```python
from build123d import *

# Parameters (mm, degrees)
SKETCH_3_R               = 5
CUT_EXTRUDE_2_DEPTH      = 151.643619181
PATTERN_CIRCULAR_1_COUNT = 4
CHAMFER_1_SIZE           = 0.5
CHAMFER_2_SIZE           = 0.5


with BuildPart() as part:
    # 草图1 → 旋转1 (revolve)
    with BuildSketch(Plane.XY, mode=Mode.PRIVATE) as revolve_1_sk:
        Polygon((0, 57.5), (0, 72.5), (38, 72.5), (38, 102.5), (53, 102.5), (53, 78), (79, 78), (79, 67.5), (63.5, 67.5), (63.5, 47.5), (58, 47.5), (58, 52.5), (45, 52.5), (45, 57.5), (5, 57.5), (5, 58.5), (3, 58.5), (3, 57.5), align=None)
    revolve(revolve_1_sk.sketch.rotate(Axis((0, 0, 0), (1, 0, 0)), 90), axis=Axis((0, 0, 0), (1, 0, 0)))

    # 草图3 → 切除-拉伸2 (cut, through all)
    with BuildSketch(Plane.ZY.offset(-38)):
        with Locations((0, 92.5)):
            Circle(SKETCH_3_R)
        with Locations((54.370135837, 74.83407198)):
            Circle(SKETCH_3_R)
        with Locations((87.972727757, 28.58407198)):
            Circle(SKETCH_3_R)
        with Locations((87.972727757, -28.58407198)):
            Circle(SKETCH_3_R)
        with Locations((54.370135837, -74.83407198)):
            Circle(SKETCH_3_R)
        with Locations((0, -92.5)):
            Circle(SKETCH_3_R)
        with Locations((-54.370135837, -74.83407198)):
            Circle(SKETCH_3_R)
        with Locations((-87.972727757, -28.58407198)):
            Circle(SKETCH_3_R)
        with Locations((-87.972727757, 28.58407198)):
            Circle(SKETCH_3_R)
        with Locations((-54.370135837, 74.83407198)):
            Circle(SKETCH_3_R)
    extrude(amount=-CUT_EXTRUDE_2_DEPTH, mode=Mode.SUBTRACT)

    # 草图5 → Ø5.0 (5) 直径孔1 (revolve, cut)
    with BuildSketch(Plane.ZX.offset(65)):
        Polygon((0, 0), (0, 16.502151548), (2.5, 15), (2.5, 0), align=None)
    hole_wizard_5_0_5_1 = revolve(axis=Axis((-6.35, 65, 0), (1, 0, 0)), mode=Mode.SUBTRACT)

    # 阵列(圆周)1: Ø5.0 (5) 直径孔1 ×4 about axis
    pattern_circular_1_axis = Axis((0, 0, 0), (1, 0, 0))
    for i in range(1, PATTERN_CIRCULAR_1_COUNT):
        add(hole_wizard_5_0_5_1.rotate(pattern_circular_1_axis, i * 360 / PATTERN_CIRCULAR_1_COUNT), mode=Mode.SUBTRACT)

    # 倒角1
    chamfer_1_edges = [part.edges().sort_by_distance(p)[0] for p in [
        (38, 0, -102.5),
        (53, 0, -102.5),
        (79, 0, -78),
        (79, 0, -67.5),
        (63.5, 0, -47.5),
        (58, 0, -47.5),
        (45, 0, -52.5),
        (0, 0, -72.5),
    ]]
    chamfer(chamfer_1_edges, length=CHAMFER_1_SIZE)

    # 倒角2
    chamfer_2_edges = [part.edges().sort_by_distance(p)[0] for p in [
        (0, -2.5, -65),
        (53, 92.5, -5),
        (38, 92.5, -5),
        (53, 74.83407198, -59.370135837),
        (38, 74.83407198, -59.370135837),
        (53, 28.58407198, -92.972727757),
        (38, 28.58407198, -92.972727757),
        (53, -28.58407198, -92.972727757),
        (38, -28.58407198, -92.972727757),
        (53, -74.83407198, -59.370135837),
        (38, -74.83407198, -59.370135837),
        (53, -92.5, -5),
        (38, -92.5, -5),
        (53, -74.83407198, 49.370135837),
        (38, -74.83407198, 49.370135837),
        (53, -28.58407198, 82.972727757),
        (38, -28.58407198, 82.972727757),
        (53, 28.58407198, 82.972727757),
        (38, 28.58407198, 82.972727757),
        (53, 74.83407198, 49.370135837),
        (38, 74.83407198, 49.370135837),
        (0, 65, -2.5),
        (0, 2.5, 65),
        (0, -65, 2.5),
    ]]
    chamfer(chamfer_2_edges, length=CHAMFER_2_SIZE)


solid = part.part
```
Geometry: final body of the model. Coordinates: model frame, mm. A direction names the side the tool comes from. Round coordinates to 2 decimals unless told otherwise and drop trailing zeros.
Item 1: Set-up query: faces 3 (the face through (63.5, -46, -16)), 4 (the face through (45, 47, -25)), 5 (the face through (45.402, 69.953, -55.454)). Return all of +Z, -Z, +X, -X, +Y, -Y with unobstructed straight access to the full face (end or side cutting, diameter ignored); none if empty.
Item 2: Pin query (flat end, axial travel): P1, Ø12, axis at x = 47, z = -55.5, coming from the +Y side; P2, Ø10, axis at y = 78.5, z = -26, coming from the +X side; P3, Ø9, axis at y = 74.83, z = 54.37, coming from the -X side; P4, Ø3, axis at y = 0, z = -65, coming from the +X side. Return the tip coordinate at first contact, or that it passes through.
Item 3: Section query A-A (z = -89). Give the number of separate pieces and of enclosed holes in the cut face, plus the area to 3 significant figures.
Item 4: Mould query, pull axis Y, two halves, no side actions, for faces 1 (the face through (45.598, 100.063, -22.22)), 2 (the face through (7.65, 1.15, -67.22)). Classes: +Y half, -Y half, draft (parallel to the pull), parting line (faces both ways), or undercut.
Item 5: Material intervals for L1, parallel to Y at x = 49, z = 2; L2, parallel to Z at x = 50, y = -26; L3, parallel to Z at x = 44, y = 2, sorted ascending.
Completed:
1. face 3: +X
1. face 4: -X
1. face 5: +X, -X
2. P1: stops at y = 89.76
2. P2: stops at x = 78.81
2. P3: passes through
2. P4: stops at x = 63.5
3. separate pieces: 3
3. enclosed holes: 0
3. area: 1,230 mm2
4. face 1: parting line
4. face 2: undercut
5. L1: y = -102.48 to -97.08, -87.92 to -52.46, 52.46 to 87.92, 97.08 to 102.48
5. L2: z = -99.15 to -92.25, -83.69 to -45.61, 45.61 to 83.69, 92.25 to 99.15
5. L3: z = -102.48 to -57.47, 57.47 to 102.48
